Design review of the part built by this model. Coordinates are the model's own, in mm. Face numbers are marked on the shaded views. A direction names the side the tool comes from. Coordinates: 2 decimals unless noted, no trailing zeros. Loops run counter-clockwise (first coordinate to the right, second up) from the corner with the lowest first, then second, coordinate; pieces in that order, holes last. Notation, with made-up numbers: (71.5, -18) -> (121.5, -18) arc R13 ccw to (121.5, 4) -> close; hole circle Ø8 at (-19.5, 40.25). An arc over 180 degrees is marked (long way). Answer in a Markdown table with one row per item.
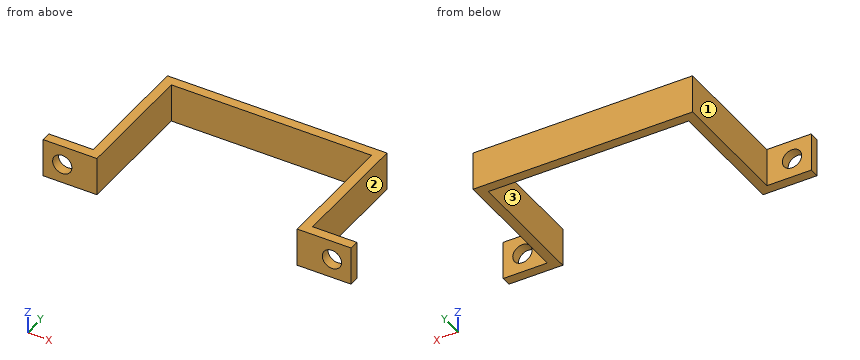
```python
from build123d import *

# Parameters (mm, degrees)
EXTRUDE_THIN1_DEPTH = 3.175
SKETCH2_R           = 1.5875
CUT_EXTRUDE1_DEPTH  = 2.54


with BuildPart() as part:
    # Sketch1 → Extrude-Thin1 (new, symmetric)
    with BuildSketch(Plane.XY):
        Polygon((-25.4, -20.574), (-16.51, -20.574), (-16.51, 0), (16.51, 0), (16.51, -20.574), (25.4, -20.574), (25.4, -18.9865), (18.0975, -18.9865), (18.0975, 1.5875), (-18.0975, 1.5875), (-18.0975, -18.9865), (-25.4, -18.9865), align=None)
    extrude(amount=EXTRUDE_THIN1_DEPTH, both=True)

    # Sketch2 → Cut-Extrude1 (cut)
    with BuildSketch(Plane(origin=(0, -18.9865, 0), x_dir=(1, 0, 0), z_dir=(0, 1, 0))):
        with Locations(Location((22.225, 0, 0), (0, 0, 270))):
            Circle(SKETCH2_R)
    cut_extrude1 = extrude(amount=-CUT_EXTRUDE1_DEPTH, mode=Mode.SUBTRACT)

    # Mirror1: Cut-Extrude1 across plane
    add(cut_extrude1.mirror(Plane(origin=(0, 0, 0), x_dir=(0, 0, 1), z_dir=(1, 0, 0))), mode=Mode.SUBTRACT)


solid = part.part
```
(1) Take a section at B-B on z = 0. Give the boundary of the cut face in (x, y).
Evaluation:
| item | result |
|---|---|
| outline | (-25.4, -20.57) -> (-23.81, -20.57) -> (-23.81, -18.99) -> (-25.4, -18.99) -> close; (-20.64, -20.57) -> (-16.51, -20.57) -> (-16.51, 0) -> (16.51, 0) -> (16.51, -20.57) -> (20.64, -20.57) -> (20.64, -18.99) -> (18.1, -18.99) -> (18.1, 1.59) -> (-18.1, 1.59) -> (-18.1, -18.99) -> (-20.64, -18.99) -> close; (23.81, -20.57) -> (25.4, -20.57) -> (25.4, -18.99) -> (23.81, -18.99) -> close |
(2) Tool access review of the marked faces 1, 2 and 3: name each direction out of +Z, -Z, +X, -X, +Y, -Y from which nothing blocks a thin tool from reaching the whole face with its end or side.
Evaluation:
| item | result |
|---|---|
| face 1 | +Z, -Z, -X, +Y |
| face 2 | +Z, -Z, +X, +Y |
| face 3 | +Z, -Z, -Y |
(3) Take a section at C-C on x = -4. Give the boundary of the cut face in (y, z) (1 decimal), and give its area (3 significant figures).
Evaluation:
| item | result |
|---|---|
| outline | (0, -3.2) -> (1.6, -3.2) -> (1.6, 3.2) -> (0, 3.2) -> close |
| area | 10.1 mm² |
(4) For pin 1 (3 mm diameter, centred on x = -6.5, z = -0.5, fed in from -Y); pin 2 (3 mm diameter, centred on y = -8, z = 1.5, fed in from +X); pin 3 (1 mm diameter, centred on y = -1, z = -2, fed in from -X); pin 4 (3 mm diameter, centred on x = -22.225, z = 0, fed in from -Y), all flat-tipped, find the tip position at first contact; note any pin that passes through.
Evaluation:
| item | result |
|---|---|
| pin 1 | stops at y = 0 |
| pin 2 | stops at x = 18.1 |
| pin 3 | stops at x = -18.1 |
| pin 4 | passes through |
(5) To check wall thickness, follow probe 1 along X at (y, z) = (-19.8, 0); probe 2 along X at (y, z) = (-10.5, 2.5); probe 3 along Y at (x, z) = (0, -1.75). State the ranges of each line that lie inside material, in increasing order.
Evaluation:
| item | result |
|---|---|
| probe 1 | x = -25.4 to -23.81, -20.64 to -16.51, 16.51 to 20.64, 23.81 to 25.4 |
| probe 2 | x = -18.1 to -16.51, 16.51 to 18.1 |
| probe 3 | y = 0 to 1.59 |
(6) Take a section at A-A on y = -11.25. Give the boundary of the cut face in (x, z) (1 decimal), and give its area (3 significant figures).
Evaluation:
| item | result |
|---|---|
| outline | (-18.1, -3.2) -> (-16.5, -3.2) -> (-16.5, 3.2) -> (-18.1, 3.2) -> close; (16.5, -3.2) -> (18.1, -3.2) -> (18.1, 3.2) -> (16.5, 3.2) -> close |
| area | 20.2 mm² |
